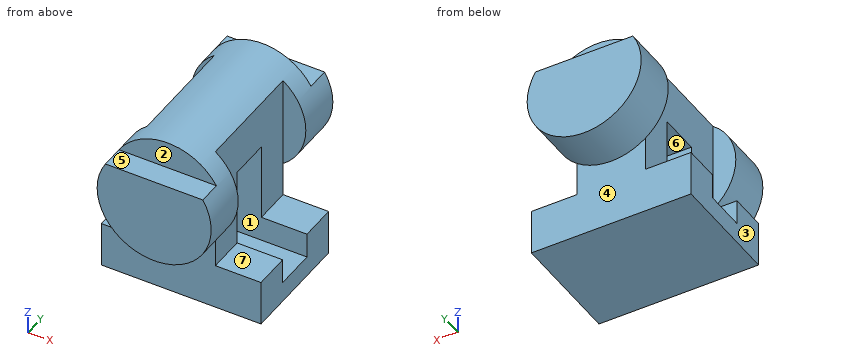
from build123d import *

# Parameters (mm, degrees)
F0_W          = 70
F0_H          = 50
F1_DEPTH      = 70
F2_R          = 25
F3_DEPTH      = 20
F3_DEPTH_BACK = 70
F4_W          = 18
F4_H          = 45
F5_DEPTH      = 70.001
F6_W          = 50
F6_H          = 20
F7_DEPTH      = 10
F8_W          = 50
F8_H          = 100
F9_DEPTH      = 20


# Not quite as in the source:
# - a pattern or mirror of a feature is missing from the dataset's text; its kind, count and spacing are read off the source's solid


with BuildPart() as f1:
    # F0 (on Top) → F1 (new body)
    with BuildSketch(Plane.XY):
        Rectangle(F0_W, F0_H)
    extrude(amount=F1_DEPTH)

    # F2 (on face) → F3 (join, two sides)
    with BuildSketch(Plane.XZ.offset(25)) as f3_sk:
        with Locations((0, 55)):
            Circle(F2_R)
    extrude(amount=F3_DEPTH)
    extrude(f3_sk.sketch, amount=-F3_DEPTH_BACK)

    # F4 (on face) → F5 (cut, through all)
    with BuildSketch(Plane.YZ.offset(35)):
        with Locations((0, 31.5)):
            Rectangle(F4_W, F4_H)
    extrude(amount=-F5_DEPTH, mode=Mode.SUBTRACT)

    # F6 (on face) → F7 (cut)
    with BuildSketch(Plane.XZ.offset(45)):
        with Locations((0, 78)):
            Rectangle(F6_W, F6_H)
    f7 = extrude(amount=-F7_DEPTH, mode=Mode.SUBTRACT)

    # F7_copies: F7 across plane
    add(f7.mirror(Plane.ZX), mode=Mode.SUBTRACT)

    # F8 (on face) → F9 (cut)
    with BuildSketch(Plane.YZ.offset(35)):
        with Locations((0, 70)):
            Rectangle(F8_W, F8_H)
    f9 = extrude(amount=-F9_DEPTH, mode=Mode.SUBTRACT)

    # F9_copies: F9 across plane
    add(f9.mirror(Plane(origin=(0, 0, 0), x_dir=(0, 0, -1), z_dir=(-1, 0, 0))), mode=Mode.SUBTRACT)


solid = f1.part
For this review, take the finished solid that the model builds, in its own axes (mm). Face numbers are marked on the shaded views. A direction names the side the tool comes from. Round coordinates to 2 decimals unless told otherwise and drop trailing zeros. Write each loop counter-clockwise with the first axis right and the second up, starting at its lowest first coordinate (ties: lowest second). Pieces come first, ordered by that corner, then holes. Notation, with made-up numbers: M 79.5,71.5 L 84.5,71.5 A31 cw 84.5,110.5 Z; hole C -17,-23.5 d4. An arc over 180 degrees is marked long. Write item = value, one per line. Start each with the question number.
(1) We need section A-A (y = 6.5). Give the boundary of the cut face in (x, z).
(2) The part is to be moulded in two halves that separate along Y. For the marked faces 1, 2, 3 and 4, say which applies: +Y half, -Y half, draft (parallel to the pull), parting line (faces both ways), or undercut.
(3) We need section D-D (x = 30). Give the boundary of the cut face in (y, z).
(4) We need section C-C (z = 52.5). Give the boundary of the cut face in (x, y), then the cut area to 3 significant figures.
(5) For line 1 along Y through (x, z) = (19, 57); line 2 along Y through (x, z) = (-30, 12); line 3 along Z through (x, y) = (29, 4), list the stretches that pass through material, from the lowest coordinate up.
(6) For the marked faces 5, 6 and 7, list the 3-axis set-ups (+Z, -Z, +X, -X, +Y, -Y) from which the entire face can be reached by the end or side of a thin tool; tool diameter is ignored.
(7) We need section B-B (x = 1). Give the boundary of the cut face in (y, z).
(8) Clearance check with flat-ended pins moving along their axes: pin 1 Ø13.5 at (x, z) = (16, 35.5) entering from +Y; pin 2 Ø10 at (y, z) = (36, 45.5) entering from -X; pin 3 Ø20 at (x, y) = (-9, -2) entering from +Z; pin 4 Ø6 at (x, y) = (-5.5, 31.5) entering from +Z. State where each tip first meets the part, or that it passes through.
Results found:
q1.outline = M -35,0 L 35,0 L 35,9 L -35,9 Z; M -15,54 L 15,54 L 15,75 A25 ccw -15,75 Z
q2.face_1 = undercut
q2.face_2 = -Y half
q2.face_3 = draft
q2.face_4 = +Y half
q3.outline = M -25,0 L 25,0 L 25,20 L 9,20 L 9,9 L -9,9 L -9,20 L -25,20 Z
q4.outline = M -24.87,-45 L 24.87,-45 L 24.87,-25 L 15,-25 L 15,-9 L -15,-9 L -15,-25 L -24.87,-25 Z; M -24.87,25 L -15,25 L -15,9 L 15,9 L 15,25 L 24.87,25 L 24.87,45 L -24.87,45 Z
q4.area = 2,950 mm²
q5.line_1 = -45 to -25, 25 to 45
q5.line_2 = -25 to -9, 9 to 25
q5.line_3 = 0 to 9
q6.face_5 = +Z, +X, -X, -Y
q6.face_6 = +X, -X
q6.face_7 = +Z, +X, +Y, -Y
q7.outline = M -45,30.02 L -25,30.02 L -25,0 L 25,0 L 25,30.02 L 45,30.02 L 45,68 L 35,68 L 35,79.98 L -35,79.98 L -35,68 L -45,68 Z; hole M -9,9 L 9,9 L 9,54 L -9,54 Z
q8.pin_1 = 45
q8.pin_2 = -24.59
q8.pin_3 = 80
q8.pin_4 = 79.87
